from build123d import *

# Parameters (mm, degrees)
F1_DEPTH = 3.175
F2_R     = 1.5875
F4_DEPTH = 3.175


with BuildPart() as f1:
    # F0 (on Front) → F1 (new body)
    with BuildSketch(Plane.XZ):
        Polygon((0, 15.08125), (0, 0), (63.5, 0), (63.5, 15.08125), (57.15, 15.08125), (57.15, 39.7002), (48.26, 39.7002), (48.26, 29.2862), (15.24, 29.2862), (15.24, 39.7002), (6.35, 39.7002), (6.35, 15.08125), align=None)
    extrude(amount=F1_DEPTH)

    # F2
    f2_edges = [f1.edges().sort_by_distance(p)[0] for p in [
        (6.35, -1.5875, 39.7002),
        (6.35, -1.5875, 15.08125),
        (0, -1.5875, 15.08125),
        (15.24, -1.5875, 39.7002),
        (48.26, -1.5875, 39.7002),
        (57.15, -1.5875, 39.7002),
        (57.15, -1.5875, 15.08125),
        (63.5, -1.5875, 15.08125),
        (48.26, -1.5875, 29.2862),
        (15.24, -1.5875, 29.2862),
    ]]
    fillet(f2_edges, radius=F2_R)

    # F3 (on face) → F4 (cut)
    with BuildSketch(Plane.XZ.offset(3.175)):
        with BuildLine():
            Line((51.59375, 5.3594), (56.35625, 5.3594))
            ThreePointArc((56.35625, 5.3594), (58.93435, 7.9375), (56.35625, 10.5156))
            Line((56.35625, 10.5156), (51.59375, 10.5156))
            ThreePointArc((51.59375, 10.5156), (49.01565, 7.9375), (51.59375, 5.3594))
        make_face()
        with BuildLine():
            Line((7.14375, 5.3594), (11.90625, 5.3594))
            ThreePointArc((11.90625, 5.3594), (14.48435, 7.9375), (11.90625, 10.5156))
            Line((11.90625, 10.5156), (7.14375, 10.5156))
            ThreePointArc((7.14375, 10.5156), (4.56565, 7.9375), (7.14375, 5.3594))
        make_face()
    extrude(amount=-F4_DEPTH, mode=Mode.SUBTRACT)


solid = f1.part
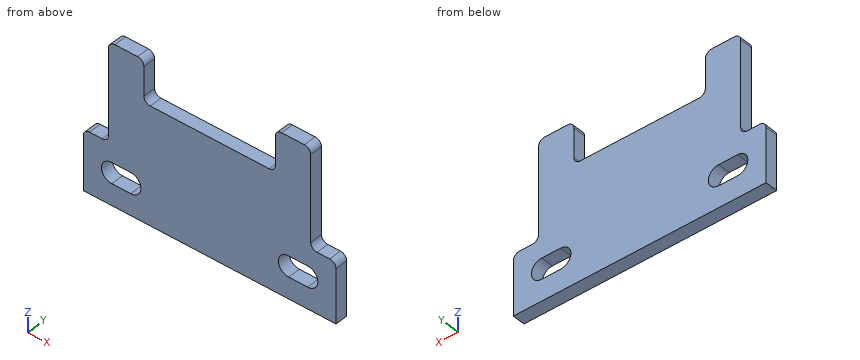
Read the model definition and answer for the solid it produces. Units are mm, in the model's axes. Round coordinates to 2 decimals unless told otherwise and drop trailing zeros. Order: outer loops, then holes, each group sorted by start corner. A loop starts at its lowest first (then second) coordinate and runs counter-clockwise, first axis right, second up.
1) Straight lines are drawn through the part: L1, parallel to X at y = -1, z = 38; L2, parallel to Z at x = 42.5, y = -1.45; L3, parallel to X at y = -2.7, z = 20. For each, find the intervals that lie inside material, in ascending order.
2) The part is cut by section A-A on z = 34. Write down the section's boundary in (x, y) (3 decimals).
3) The part is cut by section B-B on y = -0.7. Give the number of separate pieces and of enclosed holes in the cut face, plus the area to 3 significant figures.
4) The part is cut by section D-D on x = 40. Write down the section's boundary in (y, z) (3 decimals), plus the area to 3 significant figures.
5) The part is cut by section C-C on z = 21. Write down the section's boundary in (x, y) (3 decimals).
6) Flat-ended cylindrical pins translate along their axes: pin 1 (1 mm diameter, centred on x = 3.5, y = -1, fed in from +Z); pin 2 (1 mm diameter, centred on y = -1.5, z = 32.5, fed in from -X); pin 3 (1.6 mm diameter, centred on y = -1, z = 35, fed in from +X). Find the tip coordinate at first contact, or state that the pin passes through.
Resolved:
1. L1: x = 6.35 to 15.24, 48.26 to 57.15
1. L2: z = 0 to 29.29
1. L3: x = 6.35 to 57.15
2. outline: (6.35, -3.175) - (15.24, -3.175) - (15.24, 0) - (6.35, 0) - close; (48.26, -3.175) - (57.15, -3.175) - (57.15, 0) - (48.26, 0) - close
3. separate pieces: 1
3. enclosed holes: 2
3. area: 1,770 mm2
4. outline: (-3.175, 0) - (0, 0) - (0, 29.286) - (-3.175, 29.286) - close
4. area: 93.0 mm2
5. outline: (6.35, -3.175) - (57.15, -3.175) - (57.15, 0) - (6.35, 0) - close
6. pin 1: stops at z = 15.08
6. pin 2: stops at x = 6.35
6. pin 3: stops at x = 57.15
